from build123d import *

# Parameters (mm, degrees)
BOSS_EXTRUDE1_DEPTH      = 1.5875
BOSS_EXTRUDE1_DEPTH_BACK = 1.5875
SKETCH1_W                = 75
SKETCH1_H                = 60
CUT_EXTRUDE1_DEPTH       = 49.049663435
CUT_EXTRUDE1_DEPTH_BACK  = 49.049663435
SKETCH2_R                = 2.6
CUT_EXTRUDE2_DEPTH       = 49.049663435
CUT_EXTRUDE2_DEPTH_BACK  = 49.049663435
SKETCH3_R                = 6.15
SKETCH3_R_2              = 1.65


with BuildPart() as part:
    # Sketch1 → Boss-Extrude1 (new, two sides: drawn at the far end of the back side and taken through both)
    with BuildSketch(Plane(origin=(0, 0, 0), x_dir=(0, 0, -1), z_dir=(1, 0, 0)).offset(-BOSS_EXTRUDE1_DEPTH_BACK)):
        Rectangle(SKETCH1_W, SKETCH1_H)
    extrude(amount=BOSS_EXTRUDE1_DEPTH + BOSS_EXTRUDE1_DEPTH_BACK)

    # Sketch2 → Cut-Extrude1 (cut, two sides: drawn at the far end of the back side and taken through both)
    with BuildSketch(Plane(origin=(0, 0, 0), x_dir=(0, 0, -1), z_dir=(1, 0, 0)).offset(-CUT_EXTRUDE1_DEPTH_BACK)):
        with Locations((-31.05, 23.55)):
            Circle(SKETCH2_R)
        with Locations(Location((31.05, 23.55, 0), (0, 0, 180))):
            Circle(SKETCH2_R)
        with Locations((31.05, -23.55)):
            Circle(SKETCH2_R)
        with Locations(Location((-31.05, -23.55, 0), (0, 0, 180))):
            Circle(SKETCH2_R)
    extrude(amount=CUT_EXTRUDE1_DEPTH + CUT_EXTRUDE1_DEPTH_BACK, mode=Mode.SUBTRACT)

    # Sketch3 → Cut-Extrude2 (cut, two sides: drawn at the far end of the back side and taken through both)
    with BuildSketch(Plane(origin=(0, 0, 0), x_dir=(0, 0, -1), z_dir=(1, 0, 0)).offset(-CUT_EXTRUDE2_DEPTH_BACK)):
        Circle(SKETCH3_R)
        with Locations((-8.63, 8.63)):
            Circle(SKETCH3_R_2)
        with Locations(Location((-8.63, -8.63, 0), (0, 0, 180))):
            Circle(SKETCH3_R_2)
        with Locations((8.63, -8.63)):
            Circle(SKETCH3_R_2)
        with Locations(Location((8.63, 8.63, 0), (0, 0, 180))):
            Circle(SKETCH3_R_2)
    extrude(amount=CUT_EXTRUDE2_DEPTH + CUT_EXTRUDE2_DEPTH_BACK, mode=Mode.SUBTRACT)


solid = part.part
Part model, mm, in its own coordinate system. Coordinates: 2 decimals unless noted, no trailing zeros. Order: outer loops, then holes, each group sorted by start corner. A loop starts at its lowest first (then second) coordinate and runs counter-clockwise, first axis right, second up. Notation, with made-up numbers: M 82,33 L 136,33 A16 ccw 136,44 Z; hole C 59,60.25 d3. An arc over 180 degrees is marked long. Use a Markdown table: item, result.
(1) Cut at B-B on y = -8.63. Write the cut outline in (x, z), then the cut area to 3 significant figures.
A:
| item | result |
|---|---|
| outline | M -1.59,-37.5 L 1.59,-37.5 L 1.59,-10.28 L -1.59,-10.28 Z; M -1.59,-6.98 L 1.59,-6.98 L 1.59,6.98 L -1.59,6.98 Z; M -1.59,10.28 L 1.59,10.28 L 1.59,37.5 L -1.59,37.5 Z |
| area | 217 mm^2 |
(2) Cut at A-A on z = 31.05. Write the cut outline in (x, y), then the cut area to 3 significant figures.
A:
| item | result |
|---|---|
| outline | M -1.59,-30 L 1.59,-30 L 1.59,-26.15 L -1.59,-26.15 Z; M -1.59,-20.95 L 1.59,-20.95 L 1.59,20.95 L -1.59,20.95 Z; M -1.59,26.15 L 1.59,26.15 L 1.59,30 L -1.59,30 Z |
| area | 157 mm^2 |
(3) Cut at D-D on z = 0. Write the cut outline in (x, y).
A:
| item | result |
|---|---|
| outline | M -1.59,-30 L 1.59,-30 L 1.59,-6.15 L -1.59,-6.15 Z; M -1.59,6.15 L 1.59,6.15 L 1.59,30 L -1.59,30 Z |
(4) Flat gauge pins, fed straight in: pin 1 (3 mm diameter, centred on y = -23.55, z = -31.05, fed in from -X); pin 2 (6 mm diameter, centred on y = 23.55, z = -31.05, fed in from +X). Where does each tip first touch, or does it go through?
A:
| item | result |
|---|---|
| pin 1 | passes through |
| pin 2 | stops at x = 1.59 |
(5) Pull direction Y, two halves, no side cores. Call faces 1 (the cylindrical face through (-0.02, 7.24, -7.74)), 2 (the flat face through (0, 0, -37.5)), 3 (the flat face through (0, -30, 1)), 4 (the flat face through (0, 30, 1)): released by +Y, released by -Y, zero draft, split by the parting line, or undercut.
A:
| item | result |
|---|---|
| face 1 | undercut |
| face 2 | zero draft |
| face 3 | released by -Y |
| face 4 | released by +Y |
(6) Probe L1, parallel to Y at x = 0.3, z = -8.63; L2, parallel to Y at x = 0.2, z = 0; L3, parallel to Y at x = 0.25, z = 31.05. List the from-to ranges inside material, lowest first.
A:
| item | result |
|---|---|
| L1 | y = -30 to -10.28, -6.98 to 6.98, 10.28 to 30 |
| L2 | y = -30 to -6.15, 6.15 to 30 |
| L3 | y = -30 to -26.15, -20.95 to 20.95, 26.15 to 30 |
(7) Cut at C-C on x = 0.7. State how many separate pieces and enclosed holes the cut face has, then the cut area to 3 significant figures.
A:
| item | result |
|---|---|
| separate pieces | 1 |
| enclosed holes | 9 |
| area | 4,260 mm^2 |
